Autodesk Inventor part; units mm, degrees
ref_plane "YZ Plane" through (0, 0, 0) normal (1, 0, 0) x (0, 1, 0)
ref_plane "XZ Plane" through (0, 0, 0) normal (0, 1, 0) x (-1, 0, 0)
ref_plane "XY Plane" through (0, 0, 0) normal (0, 0, 1) x (1, 0, 0)
sketch "Sketch1" plane through (0, 0, 0) normal (0, 1, 0) x (-1, 0, 0)
  line L0 (0, 0) -> (8, 0)
  line L1 (8, 0) -> (8, -15)
  line L2 (8, -15) -> (0, -15)
  line L3 (0, -15) -> (0, 0)
  circle A0 centre (8, -7.5) radius 6
  point P0 (8, -13.5)
  point P1 (8, -1.5)
  dimension "d1" = 8
  dimension "d7" = 15
  dimension "d8" = 15
  dimension "d9" = 12
extrude "Extrusion1" add sketch "Sketch1" along normal blind 6 contours L0 L1 A0 L2 L3
sketch "Sketch2" plane through (0, 0, 0) normal (1, 0, 0) x (0, 0, -1)
  circle A0 centre (7.5, 3) radius 1.6
  line L0 (0, 0) -> (15, 0)
  line L1 (0, 0) -> (0, 6)
  dimension "d4" = 3.2
  dimension "d5" = 3
  dimension "d6" = 7.5
extrude "Extrusion2" cut sketch "Sketch2" against normal blind 6
properties part number "Tube_adaptor"
Part model, mm, in its own coordinate system. Round coordinates to 2 decimals unless told otherwise and drop trailing zeros. Loops run counter-clockwise (first coordinate to the right, second up) from the corner with the lowest first, then second, coordinate; pieces in that order, holes last. Notation, with made-up numbers: (-5.75, -24) -> (31.25, -24) arc R19 cw to (31.25, 4) -> close; hole circle Ø8 at (54, -5). An arc over 180 degrees is marked (long way). Use one line per item in the form item = value. Start each with the question number.
Item 1: Band-saw the part on D-D (x = -5.75). List the corners of the cut face in (y, z).
Item 2: Two-plate mould, pull along Y, no slides. Class faces 1 (the flat face through (-1, 6, -7)), 2 (the flat face through (-4, 3, 0)), 3 (the cylindrical face through (-1.09, 3.07, -5.9)), 4 (the flat face through (-1, 0, -7)): released by +Y, released by -Y, zero draft, split by the parting line, or undercut.
Item 3: Drill centre lines: line 1 along Z through (x, y) = (-1.6, 3); line 2 along Y through (x, z) = (-1.65, -7.5); line 3 along Z through (x, y) = (-3, 3.5). Where is each one in solid material? Low to high.
Item 4: Band-saw the part on A-A (y = 3). List the corners of the cut face in (x, z), plus the area to 3 significant figures.
Item 5: Band-saw the part on C-C (z = -7.5). List the corners of the cut face in (x, y), plus the area to 3 significant figures.
Item 6: Band-saw the part on B-B (x = -0.75). List the corners of the cut face in (y, z), plus the area to 3 significant figures.
Data:
q1.outline = (0, -15) -> (6, -15) -> (6, -13.06) -> (0, -13.06) -> close; (0, -1.94) -> (6, -1.94) -> (6, 0) -> (0, 0) -> close
q2.face_1 = released by +Y
q2.face_2 = zero draft
q2.face_3 = undercut
q2.face_4 = released by -Y
q3.line_1 = -15 to -9.1, -5.9 to 0
q3.line_2 = 0 to 1.4, 4.6 to 6
q3.line_3 = -15 to -10.82, -4.18 to 0
q4.outline = (-8, -15) -> (0, -15) -> (0, -9.1) -> (-2.22, -9.1) arc R6 cw to (-8, -13.5) -> close; (-8, -1.5) arc R6 cw to (-2.22, -5.9) -> (0, -5.9) -> (0, 0) -> (-8, 0) -> close
q4.area = 56.8 mm^2
q5.outline = (-2, 0) -> (0, 0) -> (0, 1.4) -> (-2, 1.4) -> close; (-2, 4.6) -> (0, 4.6) -> (0, 6) -> (-2, 6) -> close
q5.area = 5.60 mm^2
q6.outline = (0, -15) -> (6, -15) -> (6, 0) -> (0, 0) -> close; hole circle Ø3.2 at (3, -7.5)
q6.area = 82.0 mm^2
